Check sheet for the modelled part. Datum: model origin and axes. Units: mm. Give positions to 0.01 mm unless a question says otherwise; leave off trailing zeros. Order: outer loops, then holes, each group sorted by start corner. A loop starts at its lowest first (then second) coordinate and runs counter-clockwise, first axis right, second up. Notation, with made-up numbers: (46, -15.75) -> (98, -15.75) arc R13 ccw to (98, -3.75) -> close; hole circle Ø1 at (72, -18.75). An arc over 180 degrees is marked (long way). Write each question's results on one line, items separated by ' | '.
from build123d import *

# Parameters (mm, degrees)
SKETCH1_R           = 2.38125
BOSS_EXTRUDE1_DEPTH = 4.7625


with BuildPart() as part:
    # Sketch1 → Boss-Extrude1 (new body)
    with BuildSketch(Plane.XY):
        with BuildLine():
            Line((0, 9.525), (179.055725947, 9.525))
            ThreePointArc((179.055725947, 9.525), (187.345605876, -0.58786798), (177.799932549, -9.525))
            Line((177.799932549, -9.525), (0, -9.525))
            ThreePointArc((0, -9.525), (-9.525, 0), (0, 9.525))
        make_face()
        with Locations(Location((0, 0, 0), (0, 0, 180))):
            Circle(SKETCH1_R, mode=Mode.SUBTRACT)
        with Locations(Location((12.7, 0, 0), (0, 0, 180))):
            Circle(SKETCH1_R, mode=Mode.SUBTRACT)
        with Locations(Location((25.4, 0, 0), (0, 0, 180))):
            Circle(SKETCH1_R, mode=Mode.SUBTRACT)
        with Locations(Location((38.1, 0, 0), (0, 0, 180))):
            Circle(SKETCH1_R, mode=Mode.SUBTRACT)
        with Locations(Location((177.799932549, 0.041391524, 0), (0, 0, 180))):
            Circle(SKETCH1_R, mode=Mode.SUBTRACT)
        with Locations(Location((165.1, 2.22e-07, 0), (0, 0, 180))):
            Circle(SKETCH1_R, mode=Mode.SUBTRACT)
        with Locations(Location((152.4, 2.7e-08, 0), (0, 0, 180))):
            Circle(SKETCH1_R, mode=Mode.SUBTRACT)
    extrude(amount=BOSS_EXTRUDE1_DEPTH)


solid = part.part
1. Section check B-B on z = 0.75. Give the number of separate pieces and of enclosed holes in the cut face, then the cut area to 3 significant figures.
Verdict:
separate pieces: 1 | enclosed holes: 7 | area: 3,550 mm^2
2. Section check A-A on x = 12.7. Record the cut outline in (y, z) (1 decimal), then the cut area to 3 significant figures.
Verdict:
outline: (-9.5, 0) -> (-2.4, 0) -> (-2.4, 4.8) -> (-9.5, 4.8) -> close; (2.4, 0) -> (9.5, 0) -> (9.5, 4.8) -> (2.4, 4.8) -> close | area: 68.0 mm^2
3. Mould release check, pull along X, two halves, no side actions. Record for faces 1 (the flat face through (90, -9.525, 2)), 2 (the cylindrical face through (10.43, -0.72, 2.35)), 3 (the cylindrical face through (187.357, -0.387, 2.348)): +X half, -X half, draft (parallel to the pull), parting line (faces both ways), or undercut.
Verdict:
face 1: draft | face 2: undercut | face 3: +X half
4. Section check C-C on y = -6. Record the cut outline in (x, z).
Verdict:
outline: (-7.4, 0) -> (185.22, 0) -> (185.22, 4.76) -> (-7.4, 4.76) -> close
5. Gauge pin test, flat ends, axial feed: pin 1 Ø3 at (x, y) = (177.8, 0.04) entering from -Z; pin 2 Ø1 at (y, z) = (-7, 4) entering from -X. Record the tip position at first contact, or that the pin passes through.
Verdict:
pin 1: passes through | pin 2: stops at x = -6.96
6. Material ranges on probe 1 along Y at (x, z) = (12.7, 2.6) (3 decimals); probe 2 along Y at (x, z) = (25, 2.8) (3 decimals); probe 3 along X at (y, z) = (6.5, 3.85), recorded low to high. Write a range as from..to.
Verdict:
probe 1: y = -9.525..-2.381, 2.381..9.525 | probe 2: y = -9.525..-2.347, 2.347..9.525 | probe 3: x = -6.96..184.86
